```python
from build123d import *

# Parameters (mm, degrees)
F0_W     = 203.2
F0_H     = 101.6
F1_DEPTH = 101.6
F2_W     = 152.4
F2_H     = 76.2
F3_DEPTH = 76.2
F5_DEPTH = 152.4


with BuildPart() as f1:
    # F0 (on Front) → F1 (new body)
    with BuildSketch(Plane.XZ):
        with Locations((-3.343664, 13.419016)):
            Rectangle(F0_W, F0_H)
    extrude(amount=F1_DEPTH)

    # F2 (on face) → F3 (cut)
    with BuildSketch(Plane.XZ.offset(101.6)):
        with Locations((-3.343664, 26.119016)):
            Rectangle(F2_W, F2_H)
    extrude(amount=-F3_DEPTH, mode=Mode.SUBTRACT)

    # F4 (on face) → F5 (join)
    with BuildSketch(Plane.YZ.offset(-79.543664)):
        Polygon((-25.4, -11.980984), (-25.4, 64.219016), (-100.127868, -11.980984), align=None)
    extrude(amount=F5_DEPTH)


solid = f1.part
```
Here's how the part is built. I have some questions about the finished solid (model axes, mm). A direction names the side the tool comes from. Coordinates: 2 decimals unless noted, no trailing zeros. Order: outer loops, then holes, each group sorted by start corner. A loop starts at its lowest first (then second) coordinate and runs counter-clockwise, first axis right, second up. Notation, with made-up numbers: (63, 72) -> (108, 72) arc R14 cw to (108, 87) -> close; hole circle Ø3 at (27, 61.5). An arc over 180 degrees is marked (long way). Return JSON: item names as keys, results as strings.
1) If I drill on probe 1 along X at (y, z) = (-69.5, 56.5); probe 2 along Z at (x, y) = (44, -63.5); probe 3 along Y at (x, z) = (-20.5, 18.5), over which ranges is the centre line in solid material (lowest first)?
Conclusion:
{"probe 1": "x = -104.94 to -79.54, 72.86 to 98.26", "probe 2": "z = -37.38 to 25.37", "probe 3": "y = -70.24 to 0"}
2) I'm going to push flat-ended pins straight in: P1, Ø1.2, axis at x = 19.5, y = -100.5, coming from the +Z side; P2, Ø8, axis at x = 20.5, z = 1.5, coming from the -Y side; P3, Ø6, axis at x = -19.5, z = 9.5, coming from the -Y side. Where does each tip first touch, or does it pass through?
Conclusion:
{"P1": "stops at z = -11.75", "P2": "stops at y = -90.83", "P3": "stops at y = -82"}
3) If we section it at C-C on y = -41: List the corners of the cut face in (x, z) for me.
Conclusion:
{"outline": "(-104.94, -37.38) -> (98.26, -37.38) -> (98.26, 64.22) -> (72.86, 64.22) -> (72.86, 48.31) -> (-79.54, 48.31) -> (-79.54, 64.22) -> (-104.94, 64.22) -> close"}
4) If we section it at B-B on x = 15: List the corners of the cut face in (y, z) for me, plus the area to 3 significant figures.
Conclusion:
{"outline": "(-101.6, -37.38) -> (0, -37.38) -> (0, 64.22) -> (-25.4, 64.22) -> (-100.13, -11.98) -> (-101.6, -11.98) -> close", "area": "7,360 mm²"}
5) If we section it at A-A on z = 19: List the corners of the cut face in (x, y) for me, plus the area to 3 significant figures.
Conclusion:
{"outline": "(-104.94, -101.6) -> (-79.54, -101.6) -> (-79.54, -69.75) -> (72.86, -69.75) -> (72.86, -101.6) -> (98.26, -101.6) -> (98.26, 0) -> (-104.94, 0) -> close", "area": "15,800 mm²"}
6) On a 3-axis mill with a long thin cutter (end or side, diameter ignored), from which of +Z, -Z, +X, -X, +Y, -Y can I reach the whole of each face in a straight line? I mean faces 1 (the flat face through (-5, 0, 14)), 2 (the flat face through (-79.544, -73, 34)). Say none if no direction works.
Conclusion:
{"face 1": "+Z, -Z, +X, -X, +Y", "face 2": "+Z, -Y"}
7) Thinking about a two-plate mould opening in X: for faces 3 (the flat face through (-5, -50, -37.381)), 4 (the flat face through (72.856, -73, 34)), 5 (the flat face through (98.256, -50, 13)), which applies, +X half, -X half, draft (parallel to the pull), parting line (faces both ways), or undercut?
Conclusion:
{"face 3": "draft", "face 4": "undercut", "face 5": "+X half"}
